Study the drawing (mm; zero at the part's minimum x, y, z) and answer. A direction names the side the tool comes from. Round coordinates to 2 decimals unless told otherwise and drop trailing zeros. Loops run counter-clockwise (first coordinate to the right, second up) from the corner with the lowest first, then second, coordinate; pieces in that order, holes last. Notation, with made-up numbers: (48.25, 25.5) -> (85.25, 25.5) arc R25 ccw to (85.25, 46.5) -> close; hole circle Ø1 at (79, 16). An arc over 180 degrees is marked (long way). Write each question's results on one line, items separated by ' | '. Start each with the question number.
(1) The part is cut by section B-B (z = 47). Determine the outline of the cut face in (x, y).
(2) Straight lines are drawn through the part: probe 1 along Y at (x, z) = (134.5, 27); probe 2 along Z at (x, y) = (120, 10); probe 3 along Z at (x, y) = (72, 46). For each, find the intervals that lie inside material, in ascending order.
(3) Determine the mould class of the marked faces 1, 2 and 3 for opening direction Y: released by +Y, released by -Y, zero draft, split by the parting line, or undercut.
(4) The part is cut by section A-A (y = 10). Determine the outline of the cut face in (x, z), plus the area to 3 significant figures.
(5) Flat-ended cylindrical pins translate along their axes: pin 1 (2 mm diameter, centred on x = 112.5, y = 48.5, fed in from -Z); pin 2 (1.5 mm diameter, centred on x = 121, y = 18, fed in from +Z); pin 3 (3 mm diameter, centred on x = 52, y = 20, fed in from -Z); pin 4 (5.5 mm diameter, centred on x = 84.5, z = 3, fed in from +Y). Find the tip coordinate at first contact, or state that the pin passes through.
(6) The part is cut by section D-D (y = 32). Determine the outline of the cut face in (x, z).
(7) For the marked faces 4, 5, 6 and 7, determine the directions among +Z, -Z, +X, -X, +Y, -Y from which every point of the face is accessible in a straight line to the end or side of a thin tool.
(8) The part is cut by section C-C (x = 53.5). Determine the outline of the cut face in (y, z), plus the area to 3 significant figures.
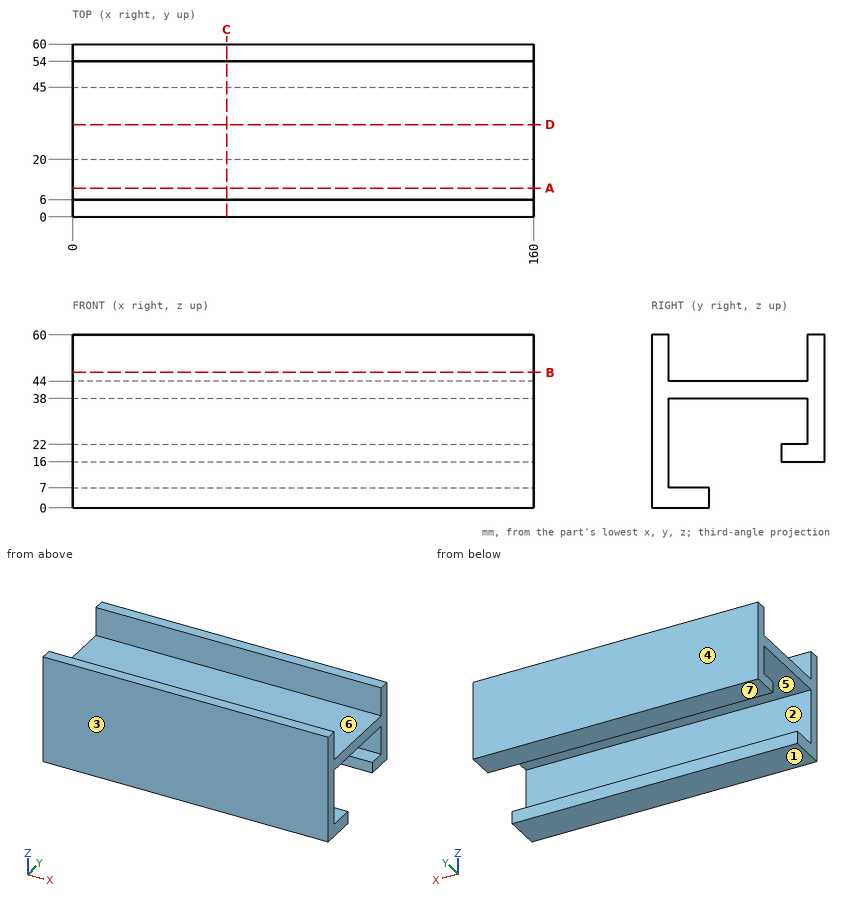
Checked values:
1) outline: (0, 0) -> (160, 0) -> (160, 6) -> (0, 6) -> close; (0, 54) -> (160, 54) -> (160, 60) -> (0, 60) -> close
2) probe 1: y = 0 to 6, 54 to 60 | probe 2: z = 0 to 7, 38 to 44 | probe 3: z = 16 to 22, 38 to 44
3) face 1: zero draft | face 2: undercut | face 3: released by -Y
4) outline: (0, 0) -> (160, 0) -> (160, 7) -> (0, 7) -> close; (0, 38) -> (160, 38) -> (160, 44) -> (0, 44) -> close | area: 2,080 mm2
5) pin 1: stops at z = 16 | pin 2: stops at z = 44 | pin 3: stops at z = 0 | pin 4: stops at y = 20
6) outline: (0, 38) -> (160, 38) -> (160, 44) -> (0, 44) -> close
7) face 4: +Z, -Z, +X, -X, +Y | face 5: +X, -X | face 6: +Z, +X, -X | face 7: -Z, +X, -X, +Y
8) outline: (0, 0) -> (20, 0) -> (20, 7) -> (6, 7) -> (6, 38) -> (54, 38) -> (54, 22) -> (45, 22) -> (45, 16) -> (60, 16) -> (60, 60) -> (54, 60) -> (54, 44) -> (6, 44) -> (6, 60) -> (0, 60) -> close | area: 1,060 mm2
